Autodesk Inventor part; units mm, degrees
ref_plane "YZ Plane" through (0, 0, 0) normal (1, 0, 0) x (0, 1, 0)
ref_plane "XZ Plane" through (0, 0, 0) normal (0, 1, 0) x (-1, 0, 0)
ref_plane "XY Plane" through (0, 0, 0) normal (0, 0, 1) x (1, 0, 0)
sketch "Sketch1" plane through (0, 0, 0) normal (0, 1, 0) x (-1, 0, 0)
  arc A0 (0, -179.3875) -> (179.3875, 0) centre (0, 0) ccw
  arc A1 (0, -134.9375) -> (134.9375, 0) centre (0, 0) ccw
  line L0 (179.3875, 0) -> (134.9375, 0)
  line L1 (0, -134.9375) -> (0, -179.3875)
  point P0 (0, -157.1625)
  point P1 (157.1625, 0)
  dimension "d0" = 179.3875
  dimension "d1" = 134.9375
extrude "Extrusion1" add sketch "Sketch1" along normal blind 0.4
sketch "Sketch2" plane through (0, 0.4, 0) normal (0, 1, 0) x (1, 0, 0)
  line L0 (-179.3875, 0) -> (-134.9375, 0)
  circle A0 centre (-143.51, 0) radius 14.2875
  point P0 (0, 0)
  dimension "d4" = 143.51
  dimension "d5" = 28.575
extrude "Extrusion2" cut sketch "Sketch2" against normal through all
fillet "Fillet1" radius 1.5875 5 edges at (-134.4823, 0.2, -11.074) (-157.7975, 0.2, 0) (-179.3875, 0.2, 0) (0, 0.2, -134.9375) (0, 0.2, -179.3875)
properties part number "3DPRINT,CABLE,GUARD" material "ABS Plastic"
Here's how the part is built. I have some questions about the finished solid (model axes, mm). Coordinates: 2 decimals unless noted, no trailing zeros. Order: outer loops, then holes, each group sorted by start corner. A loop starts at its lowest first (then second) coordinate and runs counter-clockwise, first axis right, second up.
1) Imagine slicing it at B-B on z = -38. List the corners of the cut face in (x, y) for me.
2) Imagine slicing it at A-A on x = -56. List the corners of the cut face in (y, z) for me, and give its area (3 significant figures).
3) I need wall thicknesses on line 1 (Z direction, x = -123, y = 0.15); line 2 (X direction, y = 0.2, z = -142); line 3 (X direction, y = 0.1, z = -40). Which ranges of each line are inside material? Lowest first, please.
4) We'd pull the mould along X, two halves only. Please class faces 1 (the face through (-92.025, 0.197, -98.689)), 2 (the face through (-96, 0.4, -96)), 3 (the face through (-149.96, 0.2, -12.75)): +X half, -X half, draft (parallel to the pull), parting line (faces both ways), or undercut.
Response values:
1. outline: (-175.32, 0) - (-129.48, 0) - (-129.48, 0.4) - (-175.32, 0.4) - close
2. outline: (0, -170.42) - (0.4, -170.42) - (0.4, -122.77) - (0, -122.77) - close
2. area: 19.1 mm2
3. line 1: z = -130.58 to -55.49
3. line 2: x = -109.62 to 0
3. line 3: x = -174.87 to -128.87
4. face 1: +X half
4. face 2: draft
4. face 3: undercut
